from build123d import *

# Parameters (mm, degrees)
F8_DEPTH = 32.004
F9_D     = 25.4


with BuildPart() as f8:
    # F0 (on Front) → F8 (new body)
    with BuildSketch(Plane.XZ):
        Polygon((65.036002, -37.548553), (65.036002, 37.548553), (0, 75.097106), (-65.036002, 37.548553), (-65.036002, -37.548553), (0, -75.097106), align=None)
    extrude(amount=-F8_DEPTH)

    # F9 (through all)
    with Locations(Plane.XZ):
        with Locations((-18.481843, 43.046314), (16.14237, 40.940791), (34.85816, 22.225002), (48.19316, 0), (0, -40.238947), (-30.413158, -19.183684), (-49.596842, 0), (-35.092108, 21.055264), (31.81684, -20.119473)):
            Hole(F9_D / 2)


solid = f8.part
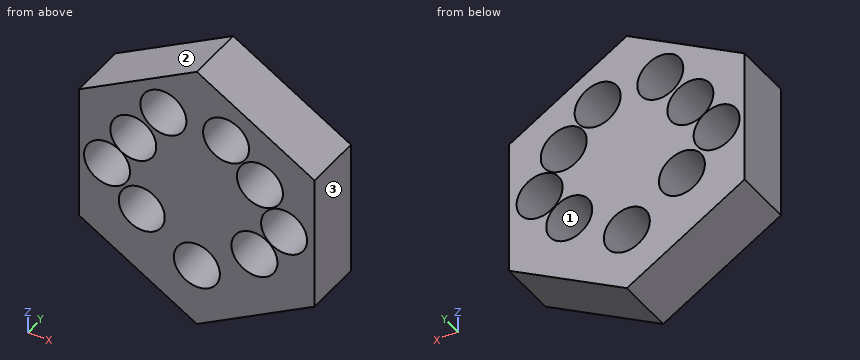
Geometry: final body of the model. Coordinates: model frame, mm. Face numbers are marked on the shaded views. Coordinates: 2 decimals unless noted, no trailing zeros. Loops run counter-clockwise (first coordinate to the right, second up) from the corner with the lowest first, then second, coordinate; pieces in that order, holes last. Notation, with made-up numbers: (-24, 37) - (21, 37) arc R23 cw to (21, 65) - close; hole circle Ø10 at (21.5, 3.5). An arc over 180 degrees is marked (long way). Put each result on its own line as item: value. Start each with the question number.
Q1. Pin query (flat end, axial travel): pin 1 Ø3 at (y, z) = (25.5, 58.5) entering from -X; pin 2 Ø23 at (x, z) = (-30.41, -19.18) entering from -Y (1 decimal); pin 3 Ø4 at (x, y) = (-29.5, 19.5) entering from -Z; pin 4 Ø1.5 at (x, y) = (-40.5, 13) entering from +Z. Return the tip coordinate at first contact, or that it passes through.
Q2. Cut plane A-A, the plane z = 0. Return loops of the section in (x, y), and give its area (3 significant figures).
Q3. Line query: line 1 (X direction, y = 28, z = -23); line 2 (X direction, y = 3, z = 49.5); line 3 (Z direction, x = -21, y = 19.5). Output: solid intervals per line, ascending.
Q4. Cut plane B-B, the plane y = 6. Give the number of separate pieces and of enclosed holes in the cut face, and give its area (3 significant figures).
Q5. Pull-direction query (X, two-part tool) for the marked faces 1, 2 and 3; classes: released by +X, released by -X, zero draft, split by the parting line, or undercut.
Filled sheet:
1. pin 1: x = -31.35
1. pin 2: through
1. pin 3: z = -59.22
1. pin 4: z = 52.15
2. outline: (-65.04, 0) - (-62.3, 0) - (-62.3, 32) - (-65.04, 32) - close; (-36.9, 0) - (35.49, 0) - (35.49, 32) - (-36.9, 32) - close; (60.89, 0) - (65.04, 0) - (65.04, 32) - (60.89, 32) - close
2. area: 2,540 mm²
3. line 1: -65.04 to -42.53, -18.3 to 19.45, 44.19 to 65.04
3. line 2: -44.34 to -29.42, -7.54 to 6.76, 25.52 to 44.34
3. line 3: -62.97 to -27.71, -10.66 to 30.6, 55.49 to 62.97
4. separate pieces: 1
4. enclosed holes: 9
4. area: 10,100 mm²
5. face 1: undercut
5. face 2: released by -X
5. face 3: released by +X
